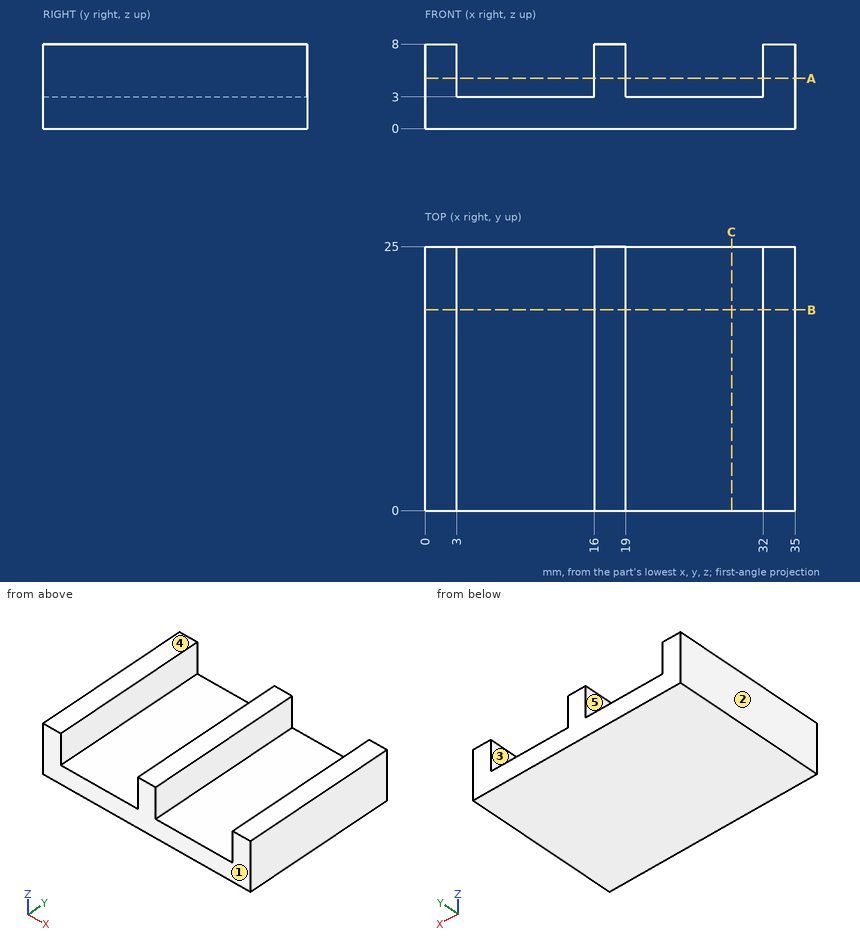
Part print with two shaded views. Sizes in mm from the minimum x, y, z corner. A direction names the side the tool comes from. Round coordinates to 2 decimals unless told otherwise and drop trailing zeros. Order: outer loops, then holes, each group sorted by start corner. A loop starts at its lowest first (then second) coordinate and runs counter-clockwise, first axis right, second up. Notation, with made-up numbers: M -17.75,-26.5 L 39.25,-26.5 A19 ccw 39.25,-4.5 Z; hole C 81,7.25 d5. An arc over 180 degrees is marked long. Use CSV: the item, a comma, the result in double quotes.
Item 1: Which spindle directions (+Z, -Z, +X, -X, +Y, -Y) get a long thin tool onto all of the face, cutting with end or side? Do the marked faces 4 and 5. Say none if no direction does.
Worked answers:
face 4,"+Z, +X, -X, +Y, -Y"
face 5,"+Z, +Y, -Y"
Item 2: Saw through at A-A (z = 4.75). List the corners of the cut face in (x, y), plus the area to 3 significant figures.
Worked answers:
outline,"M 0,0 L 3,0 L 3,25 L 0,25 Z; M 16,0 L 19,0 L 19,25 L 16,25 Z; M 32,0 L 35,0 L 35,25 L 32,25 Z"
area,"225 mm²"
Item 3: Pin check, flat tip, straight feed: pin 1 (10.5 mm diameter, centred on x = 25, y = 8, fed in from +Z). Stop position of the tip, or through.
Worked answers:
pin 1,"z = 3"
Item 4: Probe probe 1 along X at (y, z) = (5.25, 5.25); probe 2 along Z at (x, y) = (7.5, 4.5). List the from-to ranges inside material, lowest first.
Worked answers:
probe 1,"0 to 3, 16 to 19, 32 to 35"
probe 2,"0 to 3"
Item 5: Saw through at B-B (y = 19). List the corners of the cut face in (x, z).
Worked answers:
outline,"M 0,0 L 35,0 L 35,8 L 32,8 L 32,3 L 19,3 L 19,8 L 16,8 L 16,3 L 3,3 L 3,8 L 0,8 Z"
Item 6: Pull direction X, two halves, no side cores. Call the marked faces 1, 2 and 3: released by +X, released by -X, zero draft, split by the parting line, or undercut.
Worked answers:
face 1,"zero draft"
face 2,"released by -X"
face 3,"undercut"
Item 7: Saw through at C-C (x = 29). List the corners of the cut face in (y, z), plus the area to 3 significant figures.
Worked answers:
outline,"M 0,0 L 25,0 L 25,3 L 0,3 Z"
area,"75.0 mm²"
